Could you check a few things on this drawing? It's one solid part, dimensions in mm from its lowest x, y, z. A direction names the side the tool comes from. Give positions to 0.01 mm unless a question says otherwise; leave off trailing zeros. Order: outer loops, then holes, each group sorted by start corner. A loop starts at its lowest first (then second) coordinate and runs counter-clockwise, first axis right, second up. Notation, with made-up numbers: (6.5, 42) - (30.5, 42) arc R13 cw to (30.5, 57) - close; hole circle Ø7 at (27, 61). An arc over 180 degrees is marked (long way). Answer as CSV lines item,"result".
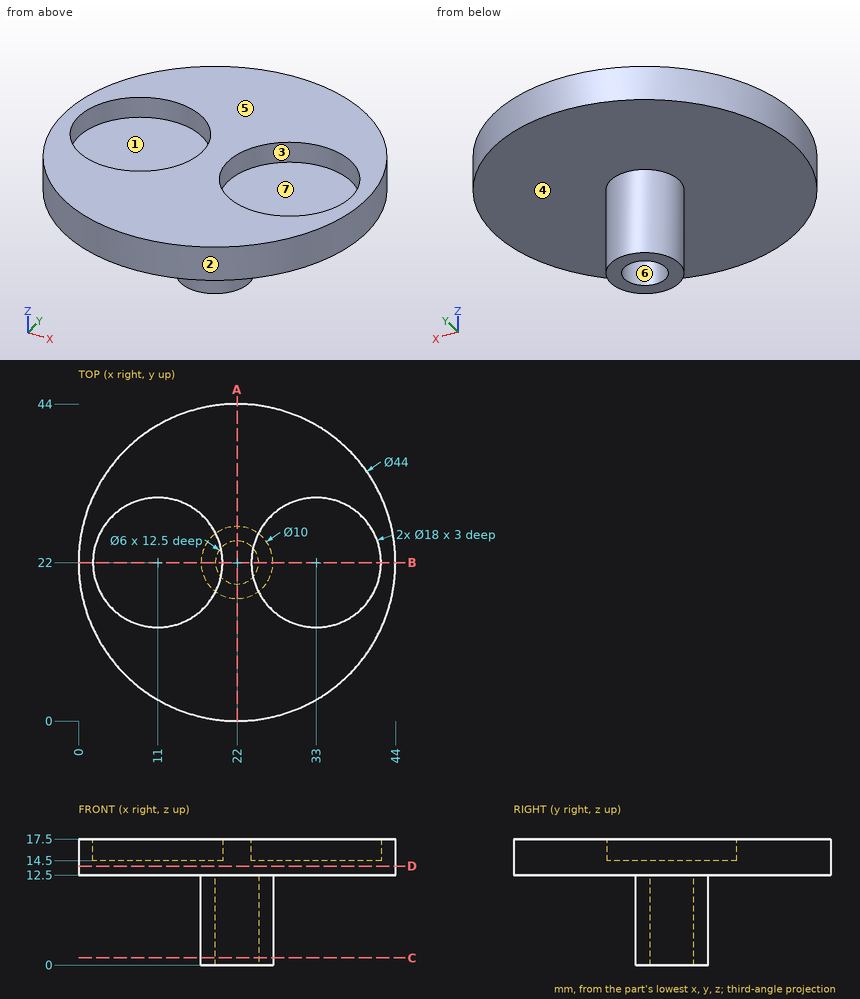
1) I'm going to push flat-ended pins straight in: P1, Ø10, axis at x = 16.5, z = 13, coming from the -Y side; P2, Ø1.8, axis at x = 21, y = 23.5, coming from the -Z side; P3, Ø4, axis at x = 31, z = 13, coming from the +Y side; P4, Ø2, axis at x = 29.5, z = 8.5, coming from the -Y side. Where does each tip first touch, or does it pass through?
Answer block:
P1,"y = 0.01"
P2,"z = 12.5"
P3,"y = 42.86"
P4,"through"
2) I want a section at B-B on y = 22. Write out the boundary of the cut face in (x, z), plus the area to 3 significant figures.
Answer block:
outline,"(0, 12.5) - (17, 12.5) - (17, 0) - (19, 0) - (19, 12.5) - (25, 12.5) - (25, 0) - (27, 0) - (27, 12.5) - (44, 12.5) - (44, 17.5) - (42, 17.5) - (42, 14.5) - (24, 14.5) - (24, 17.5) - (20, 17.5) - (20, 14.5) - (2, 14.5) - (2, 17.5) - (0, 17.5) - close"
area,"162 mm2"
3) I want a section at C-C on z = 1. Write out the boundary of the cut face in (x, y).
Answer block:
outline,"circle Ø10 at (22, 22); hole circle Ø6 at (22, 22)"
4) I want a section at D-D on z = 13.75. Write out the boundary of the cut face in (x, y), plus the area to 3 significant figures.
Answer block:
outline,"circle Ø44 at (22, 22)"
area,"1,520 mm2"
5) I need wall thicknesses on line 1 along Y through (x, z) = (22, 7.75); line 2 along Z through (x, y) = (22, 33.5); line 3 along Z through (x, y) = (35.5, 18). Which ranges of each line are inside material? Lowest first, please. Write a range as [from, to].
Answer block:
line 1,"[17, 19], [25, 27]"
line 2,"[12.5, 17.5]"
line 3,"[12.5, 14.5]"
6) If we mould it in two halves opening along X, with no side actions, what happens to the marked faces 1, 2, 3 and 4? For each: +X half, -X half, draft (parallel to the pull), parting line (faces both ways), or undercut.
Answer block:
face 1,"undercut"
face 2,"parting line"
face 3,"undercut"
face 4,"draft"
7) I want a section at A-A on x = 22. Write out the boundary of the cut face in (y, z), plus the area to 3 significant figures.
Answer block:
outline,"(0, 12.5) - (17, 12.5) - (17, 0) - (19, 0) - (19, 12.5) - (25, 12.5) - (25, 0) - (27, 0) - (27, 12.5) - (44, 12.5) - (44, 17.5) - (0, 17.5) - close"
area,"270 mm2"
8) Which directions (+Z, -Z, +X, -X, +Y, -Y) give clear straight access to the entire face, cutting with the end or side of a thin tool? Please do the marked faces 5, 6 and 7.
Answer block:
face 5,"+Z, +X, -X, +Y, -Y"
face 6,"-Z"
face 7,"+Z"
